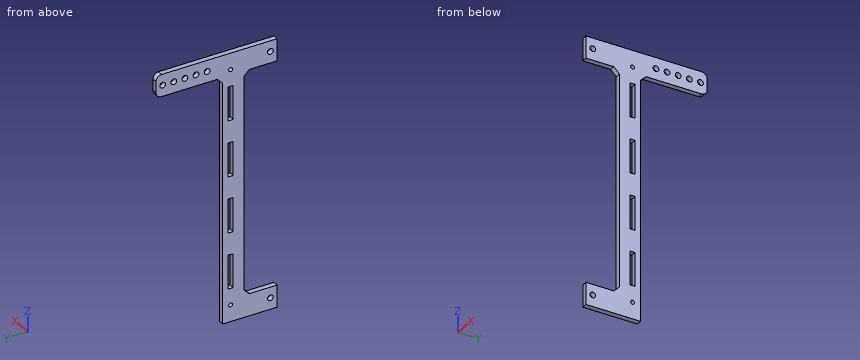
Autodesk Inventor part; units mm, degrees
ref_plane "YZ Plane" through (0, 0, 0) normal (1, 0, 0) x (0, 1, 0)
ref_plane "XZ Plane" through (0, 0, 0) normal (0, 1, 0) x (-1, 0, 0)
ref_plane "XY Plane" through (0, 0, 0) normal (0, 0, 1) x (1, 0, 0)
sketch "Sketch1" plane through (0, 0, 0) normal (1, 0, 0) x (0, 1, 0)
  line L0 (0, 0) -> (0, -38.1)
  line L1 (0, -38.1) -> (38.1, -38.1)
  line L2 (0, -308.4068) -> (0, -270.3068)
  line L3 (0, -270.3068) -> (38.1, -270.3068)
  line L4 (0, -308.4068) -> (62.1, -308.4068)
  line L5 (62.1, -308.4068) -> (62.1, -25.4)
  line L6 (62.1, -25.4) -> (138.3, -25.4)
  line L7 (138.3, -25.4) -> (138.3, 0)
  line L8 (38.1, -38.1) -> (38.1, -270.3068)
  line L9 (138.3, 0) -> (0, 0)
  line L10 (56.1, -38.1) -> (50.1, -38.1)
  line L11 (50.1, -38.1) -> (50.1, -77.1017)
  line L12 (50.1, -77.1017) -> (56.1, -77.1017)
  line L13 (56.1, -77.1017) -> (56.1, -38.1)
  line L14 (56.1, -102.5017) -> (50.1, -102.5017)
  line L15 (50.1, -102.5017) -> (50.1, -141.5034)
  line L16 (50.1, -141.5034) -> (56.1, -141.5034)
  line L17 (56.1, -141.5034) -> (56.1, -102.5017)
  line L18 (56.1, -166.9034) -> (50.1, -166.9034)
  line L19 (50.1, -166.9034) -> (50.1, -205.9051)
  line L20 (50.1, -205.9051) -> (56.1, -205.9051)
  line L21 (56.1, -205.9051) -> (56.1, -166.9034)
  line L22 (56.1, -231.3051) -> (50.1, -231.3051)
  line L23 (50.1, -231.3051) -> (50.1, -270.3068)
  line L24 (50.1, -270.3068) -> (56.1, -270.3068)
  line L25 (56.1, -270.3068) -> (56.1, -231.3051)
  point P0 (0, -289.3568)
  point P1 (56.1, -57.6008)
  point P2 (56.1, -122.0026)
  point P3 (56.1, -186.4043)
  point P4 (56.1, -250.806)
  dimension "d1" = 38.1
  dimension "d2" = 38.1
  dimension "d4" = 38.1
  dimension "d5" = 24
  dimension "d6" = 76.2
  dimension "d16" = 308.4068
  dimension "d17" = 6
  dimension "d18" = 39.0017
  dimension "d21" = 6
  dimension "d22" = 39.0017
  dimension "d23" = 25.4
  dimension "d24" = 6
  dimension "d25" = 39.0017
  dimension "d26" = 25.4
  dimension "d27" = 6
  dimension "d28" = 39.0017
  dimension "d29" = 25.4
  dimension "d49" = 25.4
  dimension "d61" = 38.1
  dimension "d62" = 50.1
extrude "Extrusion1" add sketch "Sketch1" along normal blind 6
sketch "Sketch2" plane through (0, 0, 0) normal (-1, 0, 0) x (0, 0, 1)
  circle A0 centre (-12.2165, 7.6864) radius 3.175
  circle A1 centre (-295.2013, 7.6864) radius 3.175
  point P0 (0, 0)
sketch "Sketch3" plane through (0, 0, 0) normal (-1, 0, 0) x (0, 0, 1)
  line L0 (0, 0) -> (-38.1, 0)
  line L1 (-38.1, 0) -> (-25.4, 0)
  line L2 (-25.4, 0) -> (-25.4, 38.1)
  line L3 (-25.4, 38.1) -> (-38.1, 38.1)
  line L4 (-38.1, 38.1) -> (-38.1, 0)
  line L5 (-270.3068, 38.1) -> (-270.3068, 0)
  line L6 (-270.3068, 0) -> (-283.0068, 0)
  line L7 (-283.0068, 0) -> (-283.0068, 38.1)
  line L8 (-283.0068, 38.1) -> (-270.3068, 38.1)
  line L9 (-270.3068, 38.1) -> (-270.3068, 0)
  dimension "d37" = 12.7
  dimension "d90" = 38.1
extrude "Extrusion3" cut sketch "Sketch3" against normal through all
chamfer "Chamfer1" distance 6.35 angle 45 2 edges at (3, 38.1, -283.0068) (3, 38.1, -25.4)
chamfer "Chamfer2" distance 6.35 angle 45 1 edges at (3, 62.1, -25.4)
fillet "Fillet1" radius 6.35 2 edges at (3, 138.3, -25.4) (3, 138.3, 0)
sketch "Sketch4" plane through (6, 0, 0) normal (1, 0, 0) x (0, 0, -1)
  circle A0 centre (12.7, 130.68) radius 3.175
  line L0 (19.05, 138.3) -> (6.35, 138.3)
  line L1 (25.4, 68.45) -> (25.4, 131.95)
  circle A1 centre (12.7, 117.98) radius 3.175
  circle A2 centre (12.7, 105.28) radius 3.175
  circle A3 centre (12.7, 92.58) radius 3.175
  circle A4 centre (12.7, 79.88) radius 3.175
  point P0 (0, 0)
  point P1 (12.7, 138.3)
  dimension "d50" = 6.35
  dimension "d51" = 7.62
  dimension "d54" = 12.7
sketch "Sketch5" plane through (6, 0, 0) normal (1, 0, 0) x (0, 0, -1)
  circle A0 centre (19.05, 53.1) radius 1.6256
  circle A1 centre (289.3568, 53.1) radius 1.6256
  line L0 (0, 131.95) -> (0, 0)
  line L1 (308.4068, 0) -> (308.4068, 62.1)
  line L2 (270.3068, 56.1) -> (270.3068, 50.1)
  line L3 (38.1, 50.1) -> (38.1, 56.1)
  point P0 (270.3068, 53.1)
  point P1 (38.1, 53.1)
  dimension "d63" = 3.2512
  dimension "d64" = 3.2512
  dimension "d65" = 19.05
  dimension "d66" = 19.05
hole "Hole1" at (0, 7.6864, -12.2165) at (0, 7.6864, -295.2013) direction (1, 0, 0) diameter 6.604 depth 17.0942 tip angle 118
hole "Hole2" at (6, 79.88, -12.7) at (6, 92.58, -12.7) at (6, 105.28, -12.7) at (6, 117.98, -12.7) at (6, 130.68, -12.7) direction (-1, 0, 0) diameter 6.604 depth 17.0942 tip angle 118
hole "Hole3" at (6, 53.1, -289.3568) at (6, 53.1, -19.05) direction (-1, 0, 0) diameter 4.4958 depth 17.0942 tip angle 118
properties part number "V3 Mounting Wall"
Could you check a few things on this model? Use its own coordinates, in mm. Give positions to 0.01 mm unless a question says otherwise; leave off trailing zeros. Order: outer loops, then holes, each group sorted by start corner. A loop starts at its lowest first (then second) coordinate and runs counter-clockwise, first axis right, second up.
1. Suppose I cut it at B-B (y = 79.88). List the corners of the cut face in (x, z) for me.
2. I need wall thicknesses on L1, parallel to Z at x = 1.6, y = 55.5; L2, parallel to Z at x = 3.2, y = 105; L3, parallel to Y at x = 3.4, z = -124.5. Which ranges of each line are inside material? Lowest first, please.
3. Will these pins go through, and if not, where does the flat tip stop? P1, Ø1.5, axis at x = 4.5, z = -206.5, coming from the +Y side; P2, Ø10, axis at y = 30, z = -95.5, coming from the +X side; P3, Ø1.8, axis at x = 3.5, y = 100, coming from the -Z side.
4. Suppose I cut it at C-C (z = -99.5). List the corners of the cut face in (x, y) for me, plus the area to 3 significant figures.
5. Suppose I cut it at A-A (z = -66). List the corners of the cut face in (x, y) for me, plus the area to 3 significant figures.
6. Suppose I cut it at D-D (x = 4.4). Give the number of separate pieces and of enclosed holes in the cut face, plus the area to 3 significant figures.
Solved:
1. outline: (0, -25.4) - (6, -25.4) - (6, -16) - (0, -16) - close; (0, -9.4) - (6, -9.4) - (6, 0) - (0, 0) - close
2. L1: z = -308.41 to -270.31, -231.31 to -205.91, -166.9 to -141.5, -102.5 to -77.1, -38.1 to 0
2. L2: z = -25.4 to -15.99, -9.41 to 0
2. L3: y = 38.1 to 50.1, 56.1 to 62.1
3. P1: stops at y = 62.1
3. P2: passes through
3. P3: stops at z = -25.4
4. outline: (0, 38.1) - (6, 38.1) - (6, 62.1) - (0, 62.1) - close
4. area: 144 mm2
5. outline: (0, 38.1) - (6, 38.1) - (6, 50.1) - (0, 50.1) - close; (0, 56.1) - (6, 56.1) - (6, 62.1) - (0, 62.1) - close
5. area: 108 mm2
6. separate pieces: 1
6. enclosed holes: 13
6. area: 10,100 mm2
